Could you check a few things on this model? Use its own coordinates, in mm. A direction names the side the tool comes from. Round coordinates to 2 decimals unless told otherwise and drop trailing zeros. Loops run counter-clockwise (first coordinate to the right, second up) from the corner with the lowest first, then second, coordinate; pieces in that order, holes last. Notation, with made-up numbers: M 57.25,89.5 L 61.25,89.5 A14 ccw 61.25,116.5 Z; hole C 3.25,17 d9. An arc over 180 degrees is marked long. Answer in a Markdown table with one row per item.
```python
from build123d import *

# Parameters (mm, degrees)
SWEEP1_PROFILE_R        = 16
SKETCH8_W               = 220
SKETCH8_H               = 100
BOSS_EXTRUDE1_DEPTH     = 10
BOSS_EXTRUDE3_START     = -223.510004
SKETCH12_W              = 20
SKETCH12_H              = 100
BOSS_EXTRUDE3_DEPTH     = 227.020008
SKETCH10_R              = 12.5
CUT_EXTRUDE1_DEPTH      = 17.0000001
CUT_EXTRUDE1_DEPTH_BACK = 17.0000001
SKETCH11_W              = 10
SKETCH11_H              = 50
BOSS_EXTRUDE2_DEPTH     = 36
SKETCH15_W              = 150
SKETCH15_H              = 16
BOSS_EXTRUDE4_DEPTH     = 100


with BuildPart() as part:
    # Sweep1: sweep along a path in Sketch1
    with BuildLine(Plane.XY) as sweep1_path:
        Line((-126, -59.5), (-126, 40.5))
        Line((-126, 40.5), (-126, 59.5))
        ThreePointArc((-126, 59.5), (-125.179239367, 66.4693608), (-122.761867336, 73.057376467))
        Line((-122.761867336, 73.057376467), (-47.725330083, 221.177321367))
        ThreePointArc((-47.725330083, 221.177321367), (0, 250.5), (47.725330083, 221.177321367))
        Line((47.725330083, 221.177321367), (122.761867336, 73.057376467))
        ThreePointArc((122.761867336, 73.057376467), (125.179239367, 66.4693608), (126, 59.5))
        Line((126, 59.5), (126, 40.5))
        Line((126, 40.5), (126, -59.5))
    # Sweep1 profile (on start of the path) → Sweep1 (sweep)
    with BuildSketch(Plane(origin=(-126, -59.5, 0), x_dir=(0, 0, 1), z_dir=(0, 1, 0))):
        Circle(SWEEP1_PROFILE_R)
    sweep(path=sweep1_path.line)



with BuildPart() as body_2:
    # Sketch8 → Boss-Extrude1 (new body, symmetric)
    with BuildSketch(Plane.XY):
        with Locations((0, -9.5)):
            Rectangle(SKETCH8_W, SKETCH8_H)
    extrude(amount=BOSS_EXTRUDE1_DEPTH, both=True)


with BuildPart() as part_1:
    add(part.part)

    add(body_2.part)  # Boss-Extrude3 merges body 2
    # Sketch12 → Boss-Extrude3 (add)
    with BuildSketch(Plane.ZY.offset(110).offset(BOSS_EXTRUDE3_START)):
        with Locations((0, -9.5)):
            Rectangle(SKETCH12_W, SKETCH12_H)
    extrude(amount=BOSS_EXTRUDE3_DEPTH)

    # Sketch10 → Cut-Extrude1 (cut, two sides)
    with BuildSketch(Plane.XY) as cut_extrude1_sk:
        with Locations((80, -9.5)):
            Circle(SKETCH10_R)
        with Locations((-80, -9.5)):
            Circle(SKETCH10_R)
    extrude(amount=CUT_EXTRUDE1_DEPTH, mode=Mode.SUBTRACT)
    extrude(cut_extrude1_sk.sketch, amount=-CUT_EXTRUDE1_DEPTH_BACK, mode=Mode.SUBTRACT)

    # Sketch11 → Boss-Extrude2 (add, symmetric)
    with BuildSketch(Plane.XY):
        with Locations((-100, -9.5)):
            Rectangle(SKETCH11_W, SKETCH11_H)
        with Locations((-60, -9.5)):
            Rectangle(SKETCH11_W, SKETCH11_H)
        with Locations((60, -9.5)):
            Rectangle(SKETCH11_W, SKETCH11_H)
        with Locations((100, -9.5)):
            Rectangle(SKETCH11_W, SKETCH11_H)
    extrude(amount=BOSS_EXTRUDE2_DEPTH, both=True)

    # Sketch15 → Boss-Extrude4 (add, symmetric)
    with BuildSketch(Plane(origin=(0, 0, 0), x_dir=(0, 0, -1), z_dir=(1, 0, 0))):
        with Locations((0, -67.5)):
            Rectangle(SKETCH15_W, SKETCH15_H)
    extrude(amount=BOSS_EXTRUDE4_DEPTH, both=True)


solid = part_1.part
```
1) Which directions (+Z, -Z, +X, -X, +Y, -Y) give clear straight access to the entire face, cutting with the end or side of a thin tool? Please do faces 5 (the face through (-68, -6, 0)), 6 (the face through (105, -10, 23)), 7 (the face through (-100, -9, 36)), 8 (the face through (95, -10, -23)), 9 (the face through (55, -10, 23)).
Computed:
| item | result |
|---|---|
| face 5 | +Z, -Z |
| face 6 | +Z, -Y |
| face 7 | +Z, +X, -X, +Y |
| face 8 | -Z |
| face 9 | +Z |
2) I want a section at B-B, the plane z = 29. Please give me the cut outline in (x, y), plus the area to 3 significant figures.
Computed:
| item | result |
|---|---|
| outline | M -105,-34.5 L -95,-34.5 L -95,15.5 L -105,15.5 Z; M -100,-75.5 L 100,-75.5 L 100,-59.5 L -100,-59.5 Z; M -65,-34.5 L -55,-34.5 L -55,15.5 L -65,15.5 Z; M 55,-34.5 L 65,-34.5 L 65,15.5 L 55,15.5 Z; M 95,-34.5 L 105,-34.5 L 105,15.5 L 95,15.5 Z |
| area | 5,200 mm² |
3) If we mould it in two halves opening along X, with no side actions, what happens to faces 1 (the face through (1, -68, -75)), 2 (the face through (100, -34.5, -23)), 3 (the face through (-100, -67, 1)), 4 (the face through (100, -67, 1))? For each: released by +X, released by -X, zero draft, split by the parting line, or undercut.
Computed:
| item | result |
|---|---|
| face 1 | zero draft |
| face 2 | undercut |
| face 3 | released by -X |
| face 4 | released by +X |
4) I need wall thicknesses on line 1 (X direction, y = -18.5, z = 32); line 2 (X direction, y = -9.5, z = 1); line 3 (X direction, y = -9, z = -2). Which ranges of each line are inside material? Lowest first, please.
Computed:
| item | result |
|---|---|
| line 1 | x = -105 to -95, -65 to -55, 55 to 65, 95 to 105 |
| line 2 | x = -141.97 to -92.5, -67.5 to 67.5, 92.5 to 141.97 |
| line 3 | x = -141.87 to -92.49, -67.51 to 67.51, 92.49 to 141.87 |
5) I want a section at A-A, the plane z = 0. Please give me the cut outline in (x, y).
Computed:
| item | result |
|---|---|
| outline | M -142,-59.5 L -100,-59.5 L -100,-75.5 L 100,-75.5 L 100,-59.5 L 142,-59.5 L 142,59.5 A46 ccw 137.03,80.29 L 62,228.41 A69.5 ccw -62,228.41 L -137.03,80.29 A46 ccw -142,59.5 Z; hole M -110,40.5 L 110,40.5 L 110,59.5 A14 ccw 108.49,65.83 L 33.45,213.95 A37.5 ccw -33.45,213.95 L -108.49,65.83 A14 ccw -110,59.5 Z; hole C -80,-9.5 d25; hole C 80,-9.5 d25 |
6) Will these pins go through, and if not, where does the flat tip stop? P1, Ø5, axis at x = -102.5, y = -14.5, coming from the +Z side; P2, Ø13, axis at y = 0, z = -23, coming from the -X side; P3, Ø8, axis at y = -20, z = -27.5, coming from the +X side.
Computed:
| item | result |
|---|---|
| P1 | stops at z = 36 |
| P2 | stops at x = -105 |
| P3 | stops at x = 105 |
7) I want a section at C-C, the plane y = -9.5. State how many separate pieces and enclosed holes the cut face has, plus the area to 3 significant figures.
Computed:
| item | result |
|---|---|
| separate pieces | 3 |
| enclosed holes | 0 |
| area | 7,130 mm² |
